Autodesk Inventor part; units mm, degrees
ref_plane "YZ Plane" through (0, 0, 0) normal (1, 0, 0) x (0, 1, 0)
ref_plane "XZ Plane" through (0, 0, 0) normal (0, 1, 0) x (-1, 0, 0)
ref_plane "XY Plane" through (0, 0, 0) normal (0, 0, 1) x (1, 0, 0)
sketch "スケッチ1" plane through (0, 0, 0) normal (0, 1, 0) x (-1, 0, 0)
  line L0 (0, 0) -> (30.5, 0)
  line L1 (30.5, 0) -> (30.5, -85)
  line L2 (30.5, -85) -> (0, -85)
  line L3 (0, -85) -> (0, 0)
  dimension "d0" = 30.5
  dimension "d1" = 85
extrude "押し出し1" add sketch "スケッチ1" along normal blind 3
sketch "スケッチ2" plane through (0, 3, 0) normal (0, 1, 0) x (1, 0, 0)
  line L0 (-30.5464, 15) -> (-6.0464, 15)
  line L1 (-6.0464, 15) -> (-6.0464, 70)
  line L2 (-6.0464, 70) -> (-30.5464, 70)
  line L3 (-30.5, 0) -> (0, 0)
  line L4 (-30.5464, 15) -> (-30.5464, 70)
  dimension "d4" = 24.5
  dimension "d5" = 55
  dimension "d6" = 90
  dimension "d7" = 15
extrude "押し出し2" cut sketch "スケッチ2" against normal blind 3
fillet "フィレット1" radius 2 4 edges at (-30.5, 1.5, 0) (-30.5, 1.5, -70) (-30.5, 1.5, -85) (-30.5, 1.5, -15)
fillet "フィレット2" radius 2 2 edges at (-6.0464, 1.5, -15) (-6.0464, 1.5, -70)
sketch "スケッチ3" plane through (0, 3, 0) normal (0, 1, 0) x (1, 0, 0)
  line L0 (-28.5, 0) -> (0, 0)
  line L1 (0, 0) -> (100, 0)
  line L2 (100, 0) -> (100, 85)
  line L3 (100, 85) -> (0, 85)
  line L4 (0, 85) -> (0, 0)
  dimension "d12" = 100
  dimension "d13" = 85
extrude "押し出し3" add sketch "スケッチ3" against normal blind 3
sketch "スケッチ4" plane through (0, 3, 0) normal (0, 1, 0) x (1, 0, 0)
  line L0 (100, 0) -> (100, 85)
  point P0 (0, 0)
  point P1 (40, 0)
  dimension "d16" = 60
sketch "スケッチ5" plane through (0, 3, 0) normal (0, 1, 0) x (1, 0, 0)
  line L0 (-28.5, 0) -> (100, 0)
  line L1 (39.9909, 0) -> (111.8004, 124.3777)
  line L2 (39.9909, 0) -> (183.6099, 0) construction
  line L3 (111.8004, 124.3777) -> (61.8004, 124.3777)
  line L4 (61.8004, 124.3777) -> (-28.5, 85)
  line L5 (-28.5, 85) -> (89.0656, 85)
  line L6 (100, 85) -> (-28.5, 85)
  point P0 (0, 0)
  dimension "d17" = 143.619
  dimension "d18" = 60
  dimension "d19" = 50
extrude "押し出し4" add sketch "スケッチ5" against normal blind 3
sketch "スケッチ6" plane through (0, 3, 0) normal (0, 1, 0) x (1, 0, 0)
  line L0 (111.8004, 124.3777) -> (61.8004, 124.3777)
  line L1 (111.8004, 124.3777) -> (111.8004, 0)
  line L2 (111.8004, 124.3777) -> (236.1781, 124.3777) construction
  line L3 (100, 0) -> (100, 85)
  line L4 (111.8004, 0) -> (100, 0)
  line L5 (100, 0) -> (100, 85)
  line L6 (100, 85) -> (89.0656, 85)
  line L7 (100, 85) -> (89.0656, 85)
  line L8 (89.0656, 85) -> (111.8004, 124.3777)
  line L9 (89.0656, 85) -> (111.8004, 124.3777)
  point P0 (0, 0)
  dimension "d22" = 90
extrude "押し出し5" add sketch "スケッチ6" against normal blind 3
sketch "スケッチ7" plane through (0, 3, 0) normal (0, 1, 0) x (1, 0, 0)
  line L0 (111.8004, 124.3777) -> (111.8004, 0)
  line L1 (111.8004, 109.3777) -> (39.991, 0)
  line L2 (-28.5, 0) -> (111.8004, 0)
  line L3 (111.8004, 0) -> (111.8004, 109.3777)
  line L4 (111.8004, 0) -> (39.991, 0)
  point P0 (0, 0)
  dimension "d25" = 15
extrude "押し出し6" cut sketch "スケッチ7" against normal blind 3
sketch "スケッチ8" plane through (0, 3, 0) normal (0, 1, 0) x (1, 0, 0)
  line L0 (111.8004, 109.3777) -> (111.8004, 124.3777)
  point P0 (0, 0)
  point P1 (111.8004, 116.8777)
sketch "スケッチ9" plane through (0, 3, 0) normal (0, 1, 0) x (1, 0, 0)
  point P0 (0, 0)
sketch "スケッチ10" plane through (0, 3, 0) normal (0, 1, 0) x (1, 0, 0)
  line L0 (111.8004, 109.3777) -> (39.991, 0)
  line L1 (61.8004, 124.3777) -> (111.8004, 124.3777)
  line L2 (39.991, 0) -> (111.8004, 124.3777)
  line L3 (111.8004, 109.3777) -> (111.8004, 124.3777)
  line L4 (111.8004, 124.3777) -> (111.8004, 109.3777)
  line L5 (111.8004, 109.3777) -> (39.991, 0)
  point P0 (0, 0)
extrude "押し出し7" cut sketch "スケッチ10" against normal blind 3
sketch "スケッチ11" plane through (0, 3, 0) normal (0, 1, 0) x (1, 0, 0)
  line L0 (61.8004, 124.3777) -> (74.3769, 146.1608)
  line L1 (61.8004, 124.3777) -> (86.9534, 124.3777) construction
  line L2 (74.3769, 146.1608) -> (112.1064, 124.3777)
  line L3 (111.8004, 124.3777) -> (61.8004, 124.3777)
  line L4 (112.1064, 124.3777) -> (61.8004, 124.3777)
  point P0 (0, 0)
  dimension "d32" = 25.153
  dimension "d33" = 60
extrude "押し出し8" add sketch "スケッチ11" against normal blind 3
fillet "フィレット3" radius 2 2 edges at (112.1064, 1.5, -124.3777) (111.8004, 1.5, -124.3777)
fillet "フィレット4" radius 2 3 edges at (74.3769, 1.5, -146.1608) (61.8004, 1.5, -124.3777) (39.991, 1.5, 0)
sketch "スケッチ12" plane through (0, 3, 0) normal (0, 1, 0) x (1, 0, 0)
  circle A0 centre (99.4666, 123.015) radius 1.6
  line L0 (110.1448, 125.5102) -> (76.1089, 145.1608)
  line L1 (40.5683, 1) -> (110.8769, 122.7782)
  circle A1 centre (89.4666, 128.7885) radius 1.6
  circle A2 centre (79.4666, 134.562) radius 1.6
  point P0 (0, 0)
  dimension "d38" = 3.2
  dimension "d39" = 7.5
  dimension "d40" = 10
  dimension "d41" = 3.2
  dimension "d42" = 3.2
  dimension "d43" = 10
  dimension "d44" = 7.5
  dimension "d45" = 7.5
  dimension "d46" = 10
hole "穴1" at (99.4666, 3, -123.015) at (89.4666, 3, -128.7885) at (79.4666, 3, -134.562) direction (0, -1, 0) diameter 3.2 depth 3.048
fillet "フィレット5" radius 2 1 edges at (-28.5, 1.5, -85)
sketch "スケッチ13" plane through (0, 3, 0) normal (0, 1, 0) x (1, 0, 0)
  line L0 (-30.5, 83) -> (-30.5, 72)
  line L1 (-28.1853, 85.1373) -> (61.1969, 124.1146)
  line L2 (-30.5, 83) -> (-28.1853, 85.1373)
  line L3 (-28.1853, 85.1373) -> (-30.5, 84.8107)
  arc A0 (-28.7424, 84.9853) -> (-30.5, 83) centre (-28.5, 83) ccw
  line L4 (-30.5, 84.8107) -> (-30.5, 83)
  point P0 (0, 0)
extrude "押し出し9" cut sketch "スケッチ13" against normal blind 3
fillet "フィレット6" radius 2 2 edges at (-28.1853, 1.5, -85.1373) (-30.5, 1.5, -83)
sketch "スケッチ14" plane through (0, 3, 0) normal (0, 1, 0) x (1, 0, 0)
  circle A0 centre (-20.5, 77.5) radius 1.6
  line L0 (-30.5, 82.1245) -> (-30.5, 72)
  line L1 (-28.5, 70) -> (-8.0464, 70)
  circle A1 centre (-10.5, 77.5) radius 1.6
  circle A2 centre (-0.5, 77.5) radius 1.6
  circle A3 centre (-20.5, 7.5) radius 1.6
  line L2 (-8.0464, 15) -> (-28.5, 15)
  line L3 (-30.5, 13) -> (-30.5, 2)
  circle A4 centre (-10.5, 7.5) radius 1.6
  point P0 (0, 0)
  dimension "d58" = 3.2
  dimension "d59" = 10
  dimension "d60" = 7.5
  dimension "d61" = 3.2
  dimension "d62" = 3.2
  dimension "d63" = 10
  dimension "d64" = 7.5
  dimension "d65" = 10
  dimension "d66" = 7.5
  dimension "d67" = 3.2
  dimension "d68" = 7.5
  dimension "d69" = 10
  dimension "d70" = 3.2
  dimension "d71" = 10
  dimension "d72" = 7.5
hole "穴2" at (-20.5, 3, -7.5) at (-10.5, 3, -7.5) at (-20.5, 3, -77.5) at (-10.5, 3, -77.5) at (-0.5, 3, -77.5) direction (0, -1, 0) diameter 3.2 depth 3.048
sketch "スケッチ15" plane through (0, 3, 0) normal (0, 1, 0) x (1, 0, 0)
  line L0 (32.1999, 10.4234) -> (86.628, 104.6956)
  line L1 (32.1999, 10.4234) -> (141.0561, 10.4234) construction
  line L2 (86.628, 104.6956) -> (9.117, 10.4234)
  line L3 (9.117, 10.4234) -> (32.1999, 10.4234)
  line L4 (9.117, 33.0287) -> (76.4814, 110.5538)
  line L5 (76.4814, 110.5538) -> (9.117, 63.797)
  line L6 (9.117, 63.797) -> (9.117, 33.0287)
  point P0 (0, 0)
  dimension "d80" = 60
extrude "押し出し10" cut sketch "スケッチ15" against normal blind 3
fillet "フィレット7" radius 2 6 edges at (9.117, 1.5, -63.797) (9.117, 1.5, -10.4234) (32.1999, 1.5, -10.4234) (9.117, 1.5, -33.0287) (76.4814, 1.5, -110.5538) (86.628, 1.5, -104.6956)
sketch "スケッチ16" plane through (0, 3, 0) normal (0, 1, 0) x (1, 0, 0)
  circle A0 centre (99.4666, 123.015) radius 1.6
  circle A1 centre (99.4666, 123.015) radius 1.6
  circle A2 centre (89.4666, 128.7885) radius 1.6
  circle A3 centre (89.4666, 128.7885) radius 1.6
  circle A4 centre (79.4666, 134.562) radius 1.6
  circle A5 centre (79.4666, 134.562) radius 1.6
  point P0 (0, 0)
  dimension "d84" = 3.2
  dimension "d85" = 3.2
  dimension "d86" = 3.2
extrude "押し出し11" add sketch "スケッチ16" against normal blind 3
sketch "スケッチ17" plane through (0, 3, 0) normal (0, 1, 0) x (1, 0, 0)
  circle A0 centre (99.4666, 123.015) radius 1.6
  line L0 (110.1448, 125.5102) -> (76.1089, 145.1608)
  line L1 (40.5683, 1) -> (110.8769, 122.7782)
  circle A1 centre (90.8064, 128.015) radius 1.6
  circle A2 centre (82.1461, 133.015) radius 1.6
  point P0 (0, 0)
  dimension "d89" = 3.2
  dimension "d90" = 7.5
  dimension "d91" = 10
  dimension "d92" = 3.2
  dimension "d93" = 3.2
  dimension "d95" = 7.5
  dimension "d97" = 7.5
  dimension "d98" = 20
  dimension "d99" = 30
hole "穴3" at (82.1461, 3, -133.015) at (90.8064, 3, -128.015) at (99.4666, 3, -123.015) direction (0, -1, 0) diameter 3.2 depth 3.048
equation "\"d52\" = Thickness"
equation "\"d78\" = Thickness"
equation "\"d105\" = Thickness"
equation "\"BendRadius\" = Thickness"
equation "\"BendReliefWidth\" = Thickness"
equation "\"BendReliefDepth\" = 0.5 * Thickness"
equation "\"CornerReliefSize\" = 4 * Thickness"
equation "\"MinimumRemnant\" = 2 * Thickness"
equation "\"TransitionRadius\" = BendRadius"
equation "\"JacobiRadiusSize\" = BendRadius"
equation "\"GapSize\" = Thickness"
properties part number "オムニ_前2_N"
Input: part model. Units: mm. Frame: model coordinates. A direction names the side the tool comes from. Give positions to 0.01 mm unless a question says otherwise; leave off trailing zeros. Write each loop counter-clockwise with the first axis right and the second up, starting at its lowest first coordinate (ties: lowest second). Pieces come first, ordered by that corner, then holes. Notation, with made-up numbers: (84, 10) -> (103, 10) arc R22 ccw to (103, 39) -> close; hole circle Ø2 at (87, 21.5). An arc over 180 degrees is marked (long way). Use one line per item in the form item = value. Start each with the question number.
1) Ray query, probe 1 along Z at (x, y) = (31, 2.4); probe 2 along Z at (x, y) = (-19.5, 0.35); probe 3 along X at (y, z) = (1.85, -84). Return the intervals inside material, ascending. Write a range as from..to.
2) Section query D-D on z = -112.5. Return the cut outline in (x, y).
3) Section query B-B on x = 18.5. Return the cut outline in (y, z), then the cut area to 3 significant figures.
4) Pin query (flat end, axial travel): pin 1 (1.5 mm diameter, centred on x = 60.5, y = 0.5, fed in from -Z); pin 2 (3 mm diameter, centred on x = 90.81, z = -128.01, fed in from -Y). Return the tip coordinate at first contact, or that it passes through.
5) Section query A-A on z = -25.5. Return the cut outline in (x, y), then the cut area to 3 significant figures.
6) Set-up query: faces 4 (the flat face through (39, 3, -90)), 5 (the flat face through (41.93, 1.52, -50.33)). Return all of +Z, -Z, +X, -X, +Y, -Y with unobstructed straight access to the full face (end or side cutting, diameter ignored); none if empty.
7) Draft query along Z for faces 1 (the flat face through (17.284, 1.521, -104.965)), 2 (the flat face through (53.347, 1.521, -47.05)), 3 (the flat face through (75.23, 1.521, -61.037)). Return one class per face: pulls with the +Z half, pulls with the -Z half, needs draft (parallel to the pull), parting line crosses it, or undercut.
8) Section query C-C on y = 0.85. Count the separate pieces of the cut face and the enclosed holes in it, then the cut area to 3 significant figures.
Outcome:
q1.probe_1 = -110.95..-78.99, -58.21..-37.04, -10.42..0
q1.probe_2 = -88.92..-78.75, -76.25..-70, -15..-8.75, -6.25..0
q1.probe_3 = -29.42..38.22, 53.41..69.61, 74.65..88.49
q2.outline = (34.56, 0) -> (104.94, 0) -> (104.94, 3) -> (34.56, 3) -> close
q3.outline = (0, -105.5) -> (3, -105.5) -> (3, -70.31) -> (0, -70.31) -> close; (0, -43.83) -> (3, -43.83) -> (3, -21.84) -> (0, -21.84) -> close; (0, -10.42) -> (3, -10.42) -> (3, 0) -> (0, 0) -> close
q3.area = 203 mm^2
q4.pin_1 = -124.14
q4.pin_2 = through
q5.outline = (-6.05, 0) -> (21.51, 0) -> (21.51, 3) -> (-6.05, 3) -> close; (40.9, 0) -> (54.71, 0) -> (54.71, 3) -> (40.9, 3) -> close
q5.area = 124 mm^2
q6.face_4 = +Z, -Z, +X, -X, +Y
q6.face_5 = +Y, -Y
q7.face_1 = pulls with the -Z half
q7.face_2 = undercut
q7.face_3 = pulls with the +Z half
q8.separate_pieces = 1
q8.enclosed_holes = 10
q8.area = 8,460 mm^2
